Verification items for the finished model (mm, model axes). Coordinates: 2 decimals unless noted, no trailing zeros. Write each loop counter-clockwise with the first axis right and the second up, starting at its lowest first coordinate (ties: lowest second). Pieces come first, ordered by that corner, then holes. Notation, with made-up numbers: (87.5, 10) -> (103.5, 10) arc R19 cw to (103.5, 33) -> close; hole circle Ø5 at (42.5, 85). An arc over 180 degrees is marked (long way). Answer in a Markdown table with one row per item.
```python
from build123d import *

# Parameters (mm, degrees)
SKETCH1_R           = 4
BOSS_EXTRUDE1_DEPTH = 3.175


with BuildPart() as part:
    # Sketch1 → Boss-Extrude1 (new body)
    with BuildSketch(Plane.XY):
        with BuildLine():
            Line((7.856207737, 3.175), (279.4, 3.175))
            Line((279.4, 3.175), (279.4, -3.175))
            Line((279.4, -3.175), (7.856207737, -3.175))
            ThreePointArc((7.856207737, -3.175), (6.703743885, -3.451501144), (5.802191509, -4.220805455))
            ThreePointArc((5.802191509, -4.220805455), (-7.175, 0), (5.802191509, 4.220805455))
            ThreePointArc((5.802191509, 4.220805455), (6.703743885, 3.451501144), (7.856207737, 3.175))
        make_face()
        Circle(SKETCH1_R, mode=Mode.SUBTRACT)
    extrude(amount=BOSS_EXTRUDE1_DEPTH)


solid = part.part
```
1. Thickness scan on line 1 (X direction, y = -0.25, z = 2.9); line 2 (Y direction, x = 0, z = 2.3) (3 decimals); line 3 (Y direction, x = 250, z = 2.55) (3 decimals). Record the ranges inside material, lowest first. Write a range as from..to.
Geometry says:
| item | result |
|---|---|
| line 1 | -7.17..-3.99, 3.99..279.4 |
| line 2 | -7.175..-4, 4..7.175 |
| line 3 | -3.175..3.175 |
2. Section check B-B, the plane z = 0.75. Record the boundary of the cut face in (x, y) (3 decimals), plus the area to 3 significant figures.
Geometry says:
| item | result |
|---|---|
| outline | (5.802, -4.221) arc R2.54 cw to (7.856, -3.175) -> (279.4, -3.175) -> (279.4, 3.175) -> (7.856, 3.175) arc R2.54 cw to (5.802, 4.221) arc R7.175 ccw (long way) to start; hole circle Ø8 at (0, 0) |
| area | 1,840 mm^2 |
3. Section check D-D, the plane x = 232. Record the boundary of the cut face in (y, z) (3 decimals).
Geometry says:
| item | result |
|---|---|
| outline | (-3.175, 0) -> (3.175, 0) -> (3.175, 3.175) -> (-3.175, 3.175) -> close |
4. Section check C-C, the plane y = 0. Record the boundary of the cut face in (x, z) (3 decimals).
Geometry says:
| item | result |
|---|---|
| outline | (-7.175, 0) -> (-4, 0) -> (-4, 3.175) -> (-7.175, 3.175) -> close; (4, 0) -> (279.4, 0) -> (279.4, 3.175) -> (4, 3.175) -> close |
5. Section check A-A, the plane x = 0. Record the boundary of the cut face in (y, z) (3 decimals).
Geometry says:
| item | result |
|---|---|
| outline | (-7.175, 0) -> (-4, 0) -> (-4, 3.175) -> (-7.175, 3.175) -> close; (4, 0) -> (7.175, 0) -> (7.175, 3.175) -> (4, 3.175) -> close |
6. Mould release check, pull along Y, two halves, no side actions. Record for faces 1 (the flat face through (138, -1, 3.175)), 2 (the cylindrical face through (-7.17, -0.25, 1.57)), 3 (the cylindrical face through (-0.867, -3.905, 1.565)): released by +Y, released by -Y, zero draft, split by the parting line, or undercut.
Geometry says:
| item | result |
|---|---|
| face 1 | zero draft |
| face 2 | split by the parting line |
| face 3 | undercut |
7. Depth check by flat-ended pin: P1, Ø1, axis at x = 117.5, z = 2, coming from the +Y side (3 decimals); P2, Ø8, axis at x = 61, y = 3.5, coming from the +Z side (3 decimals). Enter the tip coordinate at first touch or a pass-through.
Geometry says:
| item | result |
|---|---|
| P1 | y = 3.175 |
| P2 | z = 3.175 |
